from build123d import *

# Parameters (mm, degrees)
BOSS_EXTRUDE1_DEPTH = 35.56
CAVITY1_DEPTH       = 35.56
FILLET1_R           = 5.08


# Read off the part's stored shape, not the designer's step: Cavity1
with BuildPart() as part:
    # Sketch1 → Boss-Extrude1 (new body)
    with BuildSketch(Plane(origin=(0, 0, 0), x_dir=(1, 0, 0), z_dir=(0, 1, 0))):
        with BuildLine():
            Line((-31.526966632, -17.78), (-22.773848077, -17.78))
            ThreePointArc((-22.773848077, -17.78), (0, -28.8925), (22.773848077, -17.78))
            Line((22.773848077, -17.78), (31.526966632, -17.78))
            ThreePointArc((31.526966632, -17.78), (0, -36.195), (-31.526966632, -17.78))
        make_face()
    extrude(amount=BOSS_EXTRUDE1_DEPTH)

    # Cavity1 outline → Cavity1 (cut)
    with BuildSketch(Plane(origin=(0, 0, 0), x_dir=(1, 0, 0), z_dir=(0, 1, 0))):
        with BuildLine():
            Line((31.526966632, -17.78), (27.067689687, -17.78))
            ThreePointArc((27.067689687, -17.78), (26.576241445, -18.506529001), (26.065297512, -19.219482059))
            Line((26.065297512, -19.219482059), (29.154265611, -19.489731749))
            Line((29.154265611, -19.489731749), (24.256224025, -25.326990406))
            Line((24.256224025, -25.326990406), (23.453686354, -22.331879039))
            ThreePointArc((23.453686354, -22.331879039), (21.529414108, -24.192406932), (19.458072067, -25.887673832))
            Line((19.458072067, -25.887673832), (22.339762624, -27.032496238))
            Line((22.339762624, -27.032496238), (15.973345502, -31.219754651))
            Line((15.973345502, -31.219754651), (16.063530451, -28.120298975))
            ThreePointArc((16.063530451, -28.120298975), (13.686492406, -29.350777683), (11.215960427, -30.380758001))
            Line((11.215960427, -30.380758001), (13.648250992, -32.303964027))
            Line((13.648250992, -32.303964027), (6.348370909, -34.48940466))
            Line((6.348370909, -34.48940466), (7.323701052, -31.546023963))
            ThreePointArc((7.323701052, -31.546023963), (4.693618264, -32.043067465), (2.031472853, -32.321221249))
            Line((2.031472853, -32.321221249), (3.81, -34.861221249))
            Line((3.81, -34.861221249), (-3.81, -34.861221249))
            Line((-3.81, -34.861221249), (-2.031472853, -32.321221249))
            ThreePointArc((-2.031472853, -32.321221249), (-4.693618264, -32.043067465), (-7.323701052, -31.546023963))
            Line((-7.323701052, -31.546023963), (-6.348370909, -34.48940466))
            Line((-6.348370909, -34.48940466), (-13.648250992, -32.303964027))
            Line((-13.648250992, -32.303964027), (-11.215960427, -30.380758001))
            ThreePointArc((-11.215960427, -30.380758001), (-13.686492406, -29.350777683), (-16.063530451, -28.120298975))
            Line((-16.063530451, -28.120298975), (-15.973345502, -31.219754651))
            Line((-15.973345502, -31.219754651), (-22.339762624, -27.032496238))
            Line((-22.339762624, -27.032496238), (-19.458072067, -25.887673832))
            ThreePointArc((-19.458072067, -25.887673832), (-21.529414108, -24.192406932), (-23.453686354, -22.331879039))
            Line((-23.453686354, -22.331879039), (-24.256224025, -25.326990406))
            Line((-24.256224025, -25.326990406), (-29.154265611, -19.489731749))
            Line((-29.154265611, -19.489731749), (-26.065297512, -19.219482059))
            ThreePointArc((-26.065297512, -19.219482059), (-26.576241445, -18.506529001), (-27.067689687, -17.78))
            Line((-27.067689687, -17.78), (-31.526966632, -17.78))
            ThreePointArc((-31.526966632, -17.78), (0, -36.195), (31.526966632, -17.78))
        make_face()
    extrude(amount=CAVITY1_DEPTH, mode=Mode.SUBTRACT)

    # Fillet1
    fillet1_edges = [part.edges().sort_by_distance(p)[0] for p in [
        (-22.773848077, 17.78, 17.78),
        (22.773848077, 17.78, 17.78),
    ]]
    fillet(fillet1_edges, radius=FILLET1_R)


solid = part.part
Verification items for the finished model (mm, model axes). A direction names the side the tool comes from. Give positions to 0.01 mm unless a question says otherwise; leave off trailing zeros. Order: outer loops, then holes, each group sorted by start corner. A loop starts at its lowest first (then second) coordinate and runs counter-clockwise, first axis right, second up. Notation, with made-up numbers: M -16,3 L 38,3 A23 cw 38,42 Z; hole C 63,0 d10. An arc over 180 degrees is marked long. Answer as a JSON object with one key per item and string values. Group by question number.
1) Access from +Z, -Z, +X, -X, +Y, -Y to the whole of each face (thin tool, end or side, straight path). Record for faces 1 (the face through (20.879, 17.531, 26.452)), 2 (the face through (23.86, 17.53, 23.85)), 3 (the face through (-23.103, 18.029, 18.202)), 4 (the face through (-20.92, 17.53, 26.47)), 5 (the face through (2.908, 17.531, 33.573)).
2) Cross-section at C-C (x = 3). Enter the section's corners in (y, z), then the cut area to 3 significant figures.
3) Cross-section at D-D (z = 33.5). Enter the section's corners in (x, y).
4) Scan lines: line 1 along X through (y, z) = (6.5, 24.25); line 2 along X through (y, z) = (30, 23); line 3 along Z through (x, y) = (20.5, 8.5). Record each from-to range of solid material in increasing order. Write a range as [from, to].
5) Depth check by flat-ended pin: pin 1 Ø6 at (x, y) = (16, 10) entering from -Z; pin 2 Ø1 at (y, z) = (10.5, 30.5) entering from -X; pin 3 Ø12 at (x, y) = (-17, 31.5) entering from -Z. Enter the tip coordinate at first touch or a pass-through.
6) Mould release check, pull along X, two halves, no side actions. Record for faces 6 (the face through (-4.657, 17.531, 32.048)), 7 (the face through (26, 18, 17.78)), 8 (the face through (-2.933, 17.531, 33.609)), 9 (the face through (-26.67, 17.53, 22.45)): released by +X, released by -X, zero draft, split by the parting line, or undercut.
7) Cross-section at B-B (z = 23). Enter the section's corners in (x, y), then the cut area to 3 significant figures.
Result sheet:
{
 "1": {"face 1": "+X, +Y, -Y", "face 2": "+Z, +Y, -Y", "face 3": "-Z, +Y, -Y", "face 4": "-X, +Y, -Y", "face 5": "+Y, -Y"},
 "2": {"outline": "M 0,28.74 L 35.56,28.74 L 35.56,32.25 L 0,32.25 Z; M 0,33.7 L 35.56,33.7 L 35.56,34.86 L 0,34.86 Z", "area": "166 mm2"},
 "3": {"outline": "M -9.65,0 L -6.68,0 L -6.68,35.56 L -9.65,35.56 Z; M -2.86,0 L 2.86,0 L 2.86,35.56 L -2.86,35.56 Z; M 6.68,0 L 9.65,0 L 9.65,35.56 L 6.68,35.56 Z"},
 "4": {"line 1": "x = [-25.16, -23.97], [-21.46, -15.71], [15.71, 21.46], [23.97, 25.16]", "line 2": "x = [-26.21, -23.63], [-22.8, -17.49], [17.49, 22.8], [23.63, 26.21]", "line 3": "z = [20.36, 25.07], [26.3, 28.24]"},
 "5": {"pin 1": "stops at z = 21.77", "pin 2": "stops at x = -17.83", "pin 3": "stops at z = 18.25"},
 "6": {"face 6": "undercut", "face 7": "zero draft", "face 8": "undercut", "face 9": "released by -X"},
 "7": {"outline": "M -26.21,0 L -23.63,0 L -23.63,35.56 L -26.21,35.56 Z; M -22.8,0 L -17.49,0 L -17.49,35.56 L -22.8,35.56 Z; M 17.49,0 L 22.8,0 L 22.8,35.56 L 17.49,35.56 Z; M 23.63,0 L 26.21,0 L 26.21,35.56 L 23.63,35.56 Z", "area": "561 mm2"}
}
